Could you check a few things on this model? Use its own coordinates, in mm. Face numbers are marked on the shaded views. A direction names the side the tool comes from. Coordinates: 2 decimals unless noted, no trailing zeros. Loops run counter-clockwise (first coordinate to the right, second up) from the corner with the lowest first, then second, coordinate; pieces in that order, holes last. Notation, with made-up numbers: (56, 16.5) -> (102, 16.5) arc R15 cw to (102, 29.5) -> close; hole circle Ø10 at (-19, 77). An arc over 180 degrees is marked (long way). One line per question, with ' | ' between items.
```python
from build123d import *

# Parameters (mm, degrees)
SKETCH1_R           = 12
BOSS_EXTRUDE1_DEPTH = 2
SKETCH2_R           = 4.5
SKETCH2_R_2         = 3
BOSS_EXTRUDE2_DEPTH = 3
SKETCH3_R           = 1.5
CUT_EXTRUDE1_DEPTH  = 3
SKETCH4_R           = 4
SKETCH4_R_2         = 3
BOSS_EXTRUDE3_DEPTH = 1
SKETCH5_R           = 0.5
CUT_EXTRUDE2_DEPTH  = 2


with BuildPart() as part:
    # Sketch1 → Boss-Extrude1 (new body)
    with BuildSketch(Plane.XY):
        with Locations((-46.692941858, 3.175)):
            Circle(SKETCH1_R)
    extrude(amount=BOSS_EXTRUDE1_DEPTH)

    # Sketch2 → Boss-Extrude2 (add)
    with BuildSketch(Plane.XY.offset(2)):
        with Locations((-46.692941858, 3.175)):
            Circle(SKETCH2_R)
        with Locations((-46.692941858, 3.175)):
            Circle(SKETCH2_R_2, mode=Mode.SUBTRACT)
    extrude(amount=BOSS_EXTRUDE2_DEPTH)

    # Sketch3 → Cut-Extrude1 (cut)
    with BuildSketch(Plane.XY.offset(2)):
        with Locations((-46.692941858, 3.175)):
            Circle(SKETCH3_R)
    extrude(amount=-CUT_EXTRUDE1_DEPTH, mode=Mode.SUBTRACT)

    # Sketch4 → Boss-Extrude3 (add)
    with BuildSketch(Plane(origin=(0, 0, 0), x_dir=(-1, 0, 0), z_dir=(0, 0, -1))):
        with Locations((46.692941858, 3.175)):
            Circle(SKETCH4_R)
        with Locations((46.692941858, 3.175)):
            Circle(SKETCH4_R_2, mode=Mode.SUBTRACT)
    extrude(amount=BOSS_EXTRUDE3_DEPTH)

    # Sketch5 → Cut-Extrude2 (cut)
    with BuildSketch(Plane(origin=(0, 0, 0), x_dir=(-1, 0, 0), z_dir=(0, 0, -1))):
        with Locations((46.692941858, -4.825)):
            Circle(SKETCH5_R)
        with Locations((39.692941858, 3.175)):
            Circle(SKETCH5_R)
        with Locations((36.692941858, 3.175)):
            Circle(SKETCH5_R)
        with Locations((53.692941858, 3.175)):
            Circle(SKETCH5_R)
        with Locations((56.692941858, 3.175)):
            Circle(SKETCH5_R)
        with Locations((39.931461074, 1.363266684)):
            Circle(SKETCH5_R)
        with Locations((37.033683596, 0.586809549)):
            Circle(SKETCH5_R)
        with Locations((39.931461074, 4.986733316)):
            Circle(SKETCH5_R)
        with Locations((37.033683596, 5.763190451)):
            Circle(SKETCH5_R)
        with Locations((53.454422642, 4.986733316)):
            Circle(SKETCH5_R)
        with Locations((56.352200121, 5.763190451)):
            Circle(SKETCH5_R)
        with Locations((53.454422642, 1.363266684)):
            Circle(SKETCH5_R)
        with Locations((56.352200121, 0.586809549)):
            Circle(SKETCH5_R)
        with Locations((46.692941858, 11.175)):
            Circle(SKETCH5_R)
        with Locations((44.622389498, -4.55240661)):
            Circle(SKETCH5_R)
        with Locations((48.763494219, 10.90240661)):
            Circle(SKETCH5_R)
        with Locations((48.763494219, -4.55240661)):
            Circle(SKETCH5_R)
        with Locations((44.622389498, 10.90240661)):
            Circle(SKETCH5_R)
    extrude(amount=-CUT_EXTRUDE2_DEPTH, mode=Mode.SUBTRACT)


solid = part.part
```
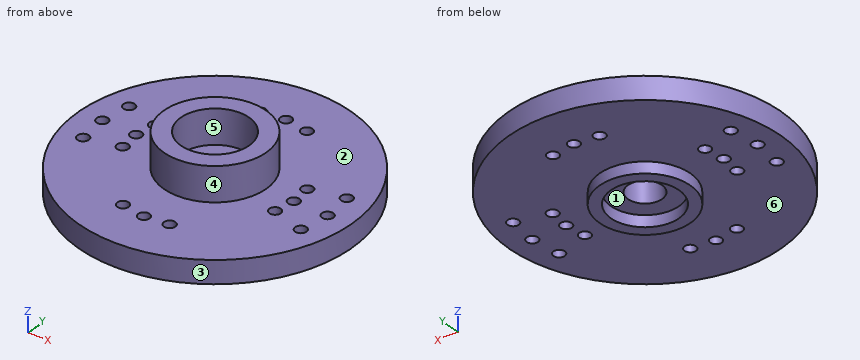
Q1. Imagine slicing it at A-A on x = -45.5. Write out the boundary of the cut face in (y, z), plus the area to 3 significant figures.
Values follow:
outline: (-8.77, 0) -> (-0.64, 0) -> (-0.64, -1) -> (0.42, -1) -> (0.42, 0) -> (2.27, 0) -> (2.27, 2) -> (0.42, 2) -> (0.42, 5) -> (-1.16, 5) -> (-1.16, 2) -> (-8.77, 2) -> close; (4.08, 0) -> (5.93, 0) -> (5.93, -1) -> (6.99, -1) -> (6.99, 0) -> (15.12, 0) -> (15.12, 2) -> (7.51, 2) -> (7.51, 5) -> (5.93, 5) -> (5.93, 2) -> (4.08, 2) -> close | area: 55.8 mm2
Q2. Imagine slicing it at B-B on z = 0.55. Give the number of separate pieces and of enclosed holes in the cut face, plus the area to 3 significant figures.
Values follow:
separate pieces: 1 | enclosed holes: 19 | area: 431 mm2
Q3. We'd pull the mould along X, two halves only. Please class the marked faces 4, 5 and 6: released by +X, released by -X, zero draft, split by the parting line, or undercut.
Values follow:
face 4: split by the parting line | face 5: undercut | face 6: zero draft
Q4. For the marked faces 1, 2 and 3, which set-ups out of +Z, -Z, +X, -X, +Y, -Y let a thin tool reach every point of the face, with its end or its side?
Values follow:
face 1: -Z | face 2: +Z | face 3: +Z, -Z
Q5. For pin 1 (5 mm diameter, centred on x = -46.69, y = 3.18, fed in from -Z); pin 2 (5.5 mm diameter, centred on x = -46.69, y = 3.18, fed in from +Z); pin 3 (2 mm diameter, centred on y = -0.5, z = 4, fed in from +X), each with a flat end and sliding along its axis, tell me the tip position at first contact or that it passes through.
Values follow:
pin 1: stops at z = 0 | pin 2: stops at z = 2 | pin 3: stops at x = -43.07
Q6. Imagine slicing it at D-D on y = -3.5. Write out the boundary of the cut face in (x, z).
Values follow:
outline: (-56.67, 0) -> (-36.72, 0) -> (-36.72, 2) -> (-56.67, 2) -> close
Q7. Please list where these lines run through material, in increasing order: L1, parallel to X at y = -4.75, z = 0.2; L2, parallel to Y at x = -46.75, z = 2.2; L3, parallel to Y at x = -48.5, z = 1.4. Write a range as [from, to].
Values follow:
L1: x = [-55.7, -49.22], [-48.3, -47.19], [-46.2, -45.08], [-44.16, -37.68] | L2: y = [-1.32, 0.18], [6.17, 7.67] | L3: y = [-8.69, -4.98], [-4.13, 10.48], [11.33, 15.04]
Q8. Imagine slicing it at C-C on x = -50. Write out the boundary of the cut face in (y, z), plus the area to 3 significant figures.
Values follow:
outline: (-8.36, 0) -> (0.92, 0) -> (0.92, -1) -> (5.43, -1) -> (5.43, 0) -> (14.71, 0) -> (14.71, 2) -> (6.23, 2) -> (6.23, 5) -> (0.12, 5) -> (0.12, 2) -> (-8.36, 2) -> close | area: 69.0 mm2
